Source: three-view drawing plus pictorial views. Frame: mm from the lowest corner of the part. Give positions to 0.01 mm unless a question says otherwise; leave off trailing zeros. Loops run counter-clockwise (first coordinate to the right, second up) from the corner with the lowest first, then second, coordinate; pieces in that order, holes last.
1. Section C-C, the plane y = 4.5. Output: boundary loops of the cut face in (x, z) (1 decimal).
2. Section A-A, the plane z = 75. Output: boundary loops of the cut face in (x, y), then the cut area to 3 significant figures.
3. Section B-B, the plane x = 75. Output: boundary loops of the cut face in (y, z), then the cut area to 3 significant figures.
4. Section D-D, the plane x = 118. Output: boundary loops of the cut face in (y, z).
5. First-contact query: P1, Ø1, axis at y = 2.5, z = 58.5, coming from the -X side; P2, Ø3, axis at y = 0.5, z = 106, coming from the +X side (1 decimal); P3, Ø3, axis at x = 117, y = 1, coming from the -Z side (1 decimal). Flat tips, straight axial feed; report the tip coordinate or a pass-through.
6. Material intervals for line 1 along X through (y, z) = (3.75, 75); line 2 along Z through (x, y) = (81.5, 3) (1 decimal); line 3 along X through (y, z) = (5.25, 82.5) (1 decimal), sorted ascending.
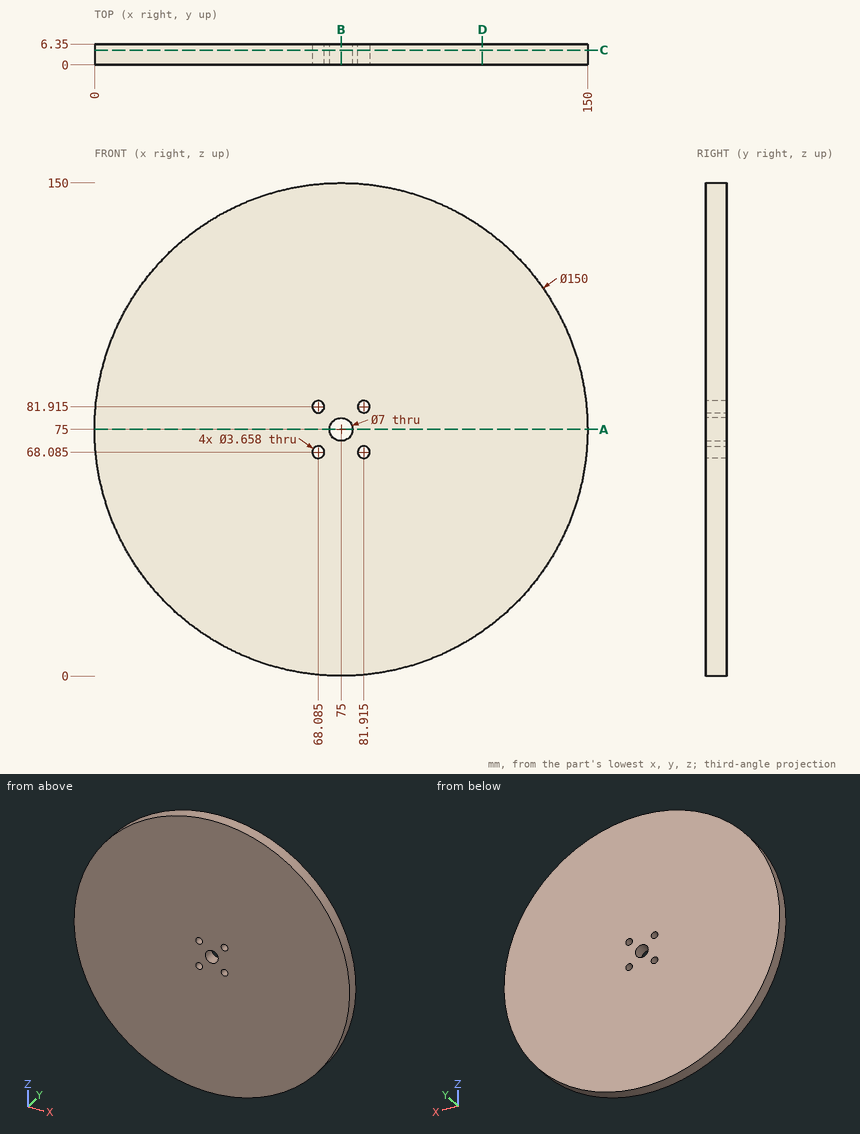
Answers below:
1. outline: circle Ø150 at (75, 75); hole circle Ø3.7 at (68.1, 68.1); hole circle Ø3.7 at (68.1, 81.9); hole circle Ø7 at (75, 75); hole circle Ø3.7 at (81.9, 68.1); hole circle Ø3.7 at (81.9, 81.9)
2. outline: (0, 0) - (71.5, 0) - (71.5, 6.35) - (0, 6.35) - close; (78.5, 0) - (150, 0) - (150, 6.35) - (78.5, 6.35) - close
2. area: 908 mm2
3. outline: (0, 0) - (6.35, 0) - (6.35, 71.5) - (0, 71.5) - close; (0, 78.5) - (6.35, 78.5) - (6.35, 150) - (0, 150) - close
3. area: 908 mm2
4. outline: (0, 13.55) - (6.35, 13.55) - (6.35, 136.45) - (0, 136.45) - close
5. P1: stops at x = 1.73
5. P2: stops at x = 144
5. P3: stops at z = 11.9
6. line 1: x = 0 to 71.5, 78.5 to 150
6. line 2: z = 0.3 to 66.3, 69.9 to 80.1, 83.7 to 149.7
6. line 3: x = 0.4 to 66.4, 69.8 to 80.2, 83.6 to 149.6
